Source: three-view drawing plus pictorial views. Frame: mm from the lowest corner of the part. Coordinates: 2 decimals unless noted, no trailing zeros. Write each loop counter-clockwise with the first axis right and the second up, starting at its lowest first coordinate (ties: lowest second). Pieces come first, ordered by that corner, then holes. Notation, with made-up numbers: (42, 82) -> (99, 82) arc R18 ccw to (99, 95) -> close; hole circle Ø4 at (-20, 39). An arc over 180 degrees is marked (long way). One line per item, written item: value.
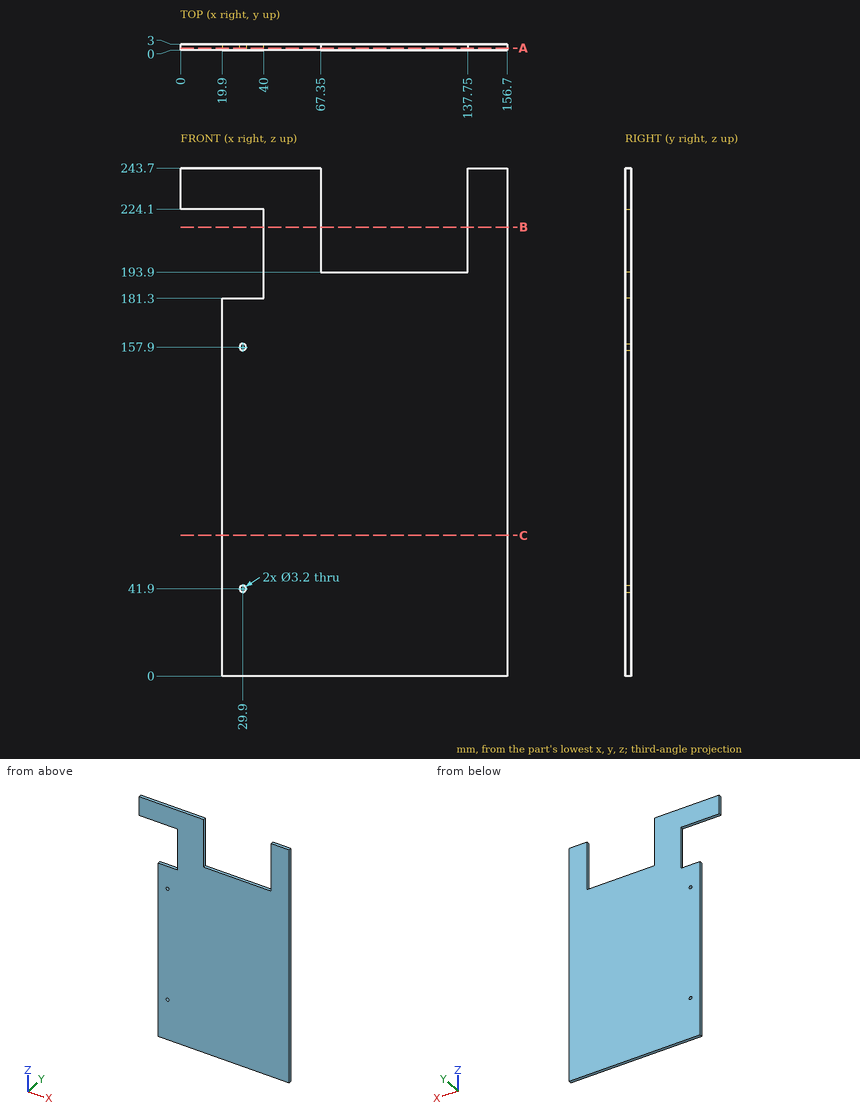
(1) Section B-B (z = 215.5). Return the cut outline in (x, y), then the cut area to 3 significant figures.
Responses:
outline: (40, 0) -> (67.35, 0) -> (67.35, 3) -> (40, 3) -> close; (137.75, 0) -> (156.7, 0) -> (156.7, 3) -> (137.75, 3) -> close
area: 139 mm2
(2) Section A-A (y = 1). Return the cut outline in (x, z).
Responses:
outline: (0, 224.1) -> (40, 224.1) -> (40, 181.3) -> (19.9, 181.3) -> (19.9, 0) -> (156.7, 0) -> (156.7, 243.7) -> (137.75, 243.7) -> (137.75, 193.9) -> (67.35, 193.9) -> (67.35, 243.7) -> (0, 243.7) -> close; hole circle Ø3.2 at (29.9, 41.9); hole circle Ø3.2 at (29.9, 157.9)
(3) Section C-C (z = 67.5). Return the cut outline in (x, y).
Responses:
outline: (19.9, 0) -> (156.7, 0) -> (156.7, 3) -> (19.9, 3) -> close
(4) First-contact query: pin 1 (0.9 mm diameter, centred on x = 13.5, y = 2, fed in from -Z); pin 2 (1 mm diameter, centred on y = 2, z = 209.5, fed in from -X); pin 3 (0.9 mm diameter, centred on y = 2, z = 130.5, fed in from -X). Flat tips, straight axial feed; report the tip coordinate or a pass-through.
Responses:
pin 1: stops at z = 224.1
pin 2: stops at x = 40
pin 3: stops at x = 19.9
(5) Line query: line 1 (Z direction, x = 29.9, y = 0.75); line 2 (X direction, y = 0.8, z = 41.9); line 3 (Z direction, x = 22, y = 1.45). Output: solid intervals per line, ascending. Write a range as [from, to].
Responses:
line 1: z = [0, 40.3], [43.5, 156.3], [159.5, 181.3], [224.1, 243.7]
line 2: x = [19.9, 28.3], [31.5, 156.7]
line 3: z = [0, 181.3], [224.1, 243.7]
